```python
from build123d import *

# Parameters (mm, degrees)
SKETCH1_W           = 533.4
SKETCH1_H           = 100
SKETCH1_R           = 1.9842329
SKETCH1_R_2         = 2.018120645
SKETCH1_R_3         = 2.032
SKETCH1_W_2         = 76.2
SKETCH1_H_2         = 6.35
SKETCH1_W_3         = 25.4
SKETCH1_W_4         = 6.35
SKETCH1_H_3         = 12.7
SKETCH1_W_5         = 38.1
BOSS_EXTRUDE1_DEPTH = 6.35
SKETCH2_R           = 1.984375
SKETCH2_R_2         = 28.360038464
SKETCH2_W           = 4.7625
SKETCH2_H           = 10.2
SKETCH2_W_2         = 10.2
SKETCH2_H_2         = 4.7625
CUT_EXTRUDE2_DEPTH  = 6.35


with BuildPart() as part:
    # Sketch1 → Boss-Extrude1 (new body)
    with BuildSketch(Plane(origin=(0, 0, 0), x_dir=(1, 0, 0), z_dir=(0, 1, 0))):
        Rectangle(SKETCH1_W, SKETCH1_H)
        with Locations((-113.583722144, -34.925)):
            Circle(SKETCH1_R, mode=Mode.SUBTRACT)
        with Locations((114.309932521, 34.925)):
            Circle(SKETCH1_R_2, mode=Mode.SUBTRACT)
        with Locations((114.309932521, -34.925)):
            Circle(SKETCH1_R_2, mode=Mode.SUBTRACT)
        with Locations((-113.583722144, 34.925)):
            Circle(SKETCH1_R, mode=Mode.SUBTRACT)
        with Locations((-55.5625, 0)):
            Circle(SKETCH1_R_3, mode=Mode.SUBTRACT)
        with Locations((55.5625, 0)):
            Circle(SKETCH1_R_3, mode=Mode.SUBTRACT)
        with Locations((0, -17.5895)):
            Circle(SKETCH1_R_3, mode=Mode.SUBTRACT)
        Rectangle(SKETCH1_W_2, SKETCH1_H_2, mode=Mode.SUBTRACT)
        with Locations((114.3, 0)):
            Rectangle(SKETCH1_W_3, SKETCH1_H_2, mode=Mode.SUBTRACT)
        with Locations((-114.3, 0)):
            Rectangle(SKETCH1_W_3, SKETCH1_H_2, mode=Mode.SUBTRACT)
        with Locations((76.2, -31.75)):
            Rectangle(SKETCH1_W_4, SKETCH1_H_3, mode=Mode.SUBTRACT)
        with Locations((-76.2, -31.75)):
            Rectangle(SKETCH1_W_4, SKETCH1_H_3, mode=Mode.SUBTRACT)
        with Locations((76.2, 31.75)):
            Rectangle(SKETCH1_W_4, SKETCH1_H_3, mode=Mode.SUBTRACT)
        with Locations((-76.2, 31.75)):
            Rectangle(SKETCH1_W_4, SKETCH1_H_3, mode=Mode.SUBTRACT)
        with Locations((184.513105188, -34.925)):
            Rectangle(SKETCH1_W_5, SKETCH1_H_2, mode=Mode.SUBTRACT)
        with Locations((-183.786894812, 34.925)):
            Rectangle(SKETCH1_W_5, SKETCH1_H_2, mode=Mode.SUBTRACT)
        with Locations((184.513105188, 34.925)):
            Rectangle(SKETCH1_W_5, SKETCH1_H_2, mode=Mode.SUBTRACT)
        with Locations((-183.786894812, -34.925)):
            Rectangle(SKETCH1_W_5, SKETCH1_H_2, mode=Mode.SUBTRACT)
        with BuildLine():
            Line((-16.279001812, 31.75), (16.279001812, 31.75))
            ThreePointArc((16.279001812, 31.75), (0, 6.82), (-16.279001812, 31.75))
        make_face(mode=Mode.SUBTRACT)
    extrude(amount=BOSS_EXTRUDE1_DEPTH)

    # Sketch2 → Cut-Extrude2 (cut)
    with BuildSketch(Plane(origin=(0, 0, 0), x_dir=(1, 0, 0), z_dir=(0, 1, 0))):
        with Locations((-169.08125, 22)):
            Circle(SKETCH2_R)
        with Locations((-169.08125, -22)):
            Circle(SKETCH2_R)
        with Locations((-194.7, -47.61875)):
            Circle(SKETCH2_R)
        with Locations((-238.7, -47.61875)):
            Circle(SKETCH2_R)
        with Locations((-264.31875, -22)):
            Circle(SKETCH2_R)
        with Locations((-264.31875, 22)):
            Circle(SKETCH2_R)
        with Locations((-194.7, 47.61875)):
            Circle(SKETCH2_R)
        with Locations((-238.7, 47.61875)):
            Circle(SKETCH2_R)
        with Locations((-216.7, 0)):
            Circle(SKETCH2_R_2)
        with Locations((216.7, 0)):
            Circle(SKETCH2_R_2)
        with Locations((238.7, 47.61875)):
            Circle(SKETCH2_R)
        with Locations((194.7, 47.61875)):
            Circle(SKETCH2_R)
        with Locations((264.31875, 22)):
            Circle(SKETCH2_R)
        with Locations((264.31875, -22)):
            Circle(SKETCH2_R)
        with Locations((238.7, -47.61875)):
            Circle(SKETCH2_R)
        with Locations((194.7, -47.61875)):
            Circle(SKETCH2_R)
        with Locations((169.08125, -22)):
            Circle(SKETCH2_R)
        with Locations((169.08125, 22)):
            Circle(SKETCH2_R)
        with Locations((-169.08125, 0)):
            Rectangle(SKETCH2_W, SKETCH2_H)
        with Locations((-264.31875, 0)):
            Rectangle(SKETCH2_W, SKETCH2_H)
        with Locations((-216.7, 47.61875)):
            Rectangle(SKETCH2_W_2, SKETCH2_H_2)
        with Locations((-216.7, -47.61875)):
            Rectangle(SKETCH2_W_2, SKETCH2_H_2)
        with Locations((216.7, -47.61875)):
            Rectangle(SKETCH2_W_2, SKETCH2_H_2)
        with Locations((216.7, 47.61875)):
            Rectangle(SKETCH2_W_2, SKETCH2_H_2)
        with Locations((264.31875, 0)):
            Rectangle(SKETCH2_W, SKETCH2_H)
        with Locations((169.08125, 0)):
            Rectangle(SKETCH2_W, SKETCH2_H)
    extrude(amount=CUT_EXTRUDE2_DEPTH, mode=Mode.SUBTRACT)


solid = part.part
```
Read the model definition and answer for the solid it produces. Units are mm, in the model's axes. Give positions to 0.01 mm unless a question says otherwise; leave off trailing zeros. Write each loop counter-clockwise with the first axis right and the second up, starting at its lowest first coordinate (ties: lowest second). Pieces come first, ordered by that corner, then holes. Notation, with made-up numbers: (8.25, -36.5) -> (35.25, -36.5) arc R32 ccw to (35.25, -3.5) -> close; hole circle Ø1 at (-34, -6.5). An arc over 180 degrees is marked (long way). Answer as a JSON object with one key per item and string values.
1) Section B-B on x = 106 is taken. Write down the section's boundary in (y, z) (3 decimals).
Findings below:
{"outline": "(0, -50) -> (6.35, -50) -> (6.35, -3.175) -> (0, -3.175) -> close; (0, 3.175) -> (6.35, 3.175) -> (6.35, 50) -> (0, 50) -> close"}
2) Straight lines are drawn through the part: probe 1 along Z at (x, y) = (216.7, 4.75); probe 2 along X at (y, z) = (1.75, -38) (3 decimals); probe 3 along Z at (x, y) = (-240.5, 5.5). For each, find the intervals that lie inside material, in ascending order. Write a range as from..to.
Findings below:
{"probe 1": "z = -45.24..-28.36, 28.36..45.24", "probe 2": "x = -266.7..-202.837, -164.737..-79.375, -73.025..73.025, 79.375..165.463, 203.563..266.7", "probe 3": "z = -50..-48.45, -46.78..-15.42, 15.42..46.78, 48.45..50"}
3) For a pull along X with two mould halves and no side action, classify faces 1 (the cylindrical face through (0.494, 3.131, -6.827)), 2 (the flat face through (-4, 0, 10)) as pulls with the +X half, pulls with the -X half, needs draft (parallel to the pull), parting line crosses it, or undercut.
Findings below:
{"face 1": "undercut", "face 2": "needs draft"}
4) Section A-A on x = 216.7 is taken. Write down the section's boundary in (y, z), then the cut area to 3 significant figures.
Findings below:
{"outline": "(0, -45.24) -> (6.35, -45.24) -> (6.35, -28.36) -> (0, -28.36) -> close; (0, 28.36) -> (6.35, 28.36) -> (6.35, 45.24) -> (0, 45.24) -> close", "area": "214 mm^2"}
5) Section C-C on y = 5 is taken. Count the separate pieces of the cut face and the enclosed holes in it, then the cut area to 3 significant figures.
Findings below:
{"separate pieces": "1", "enclosed holes": "39", "area": "44,800 mm^2"}
